Source: three-view drawing plus pictorial views. Frame: mm from the lowest corner of the part. A direction names the side the tool comes from. Give positions to 0.01 mm unless a question says otherwise; leave off trailing zeros. Loops run counter-clockwise (first coordinate to the right, second up) from the corner with the lowest first, then second, coordinate; pieces in that order, holes last. Notation, with made-up numbers: (43.25, -30) -> (68.25, -30) arc R19 cw to (68.25, 4) -> close; hole circle Ø7 at (14.5, 10). An arc over 180 degrees is marked (long way). Answer in a Markdown table with one row per item. Add a question column.
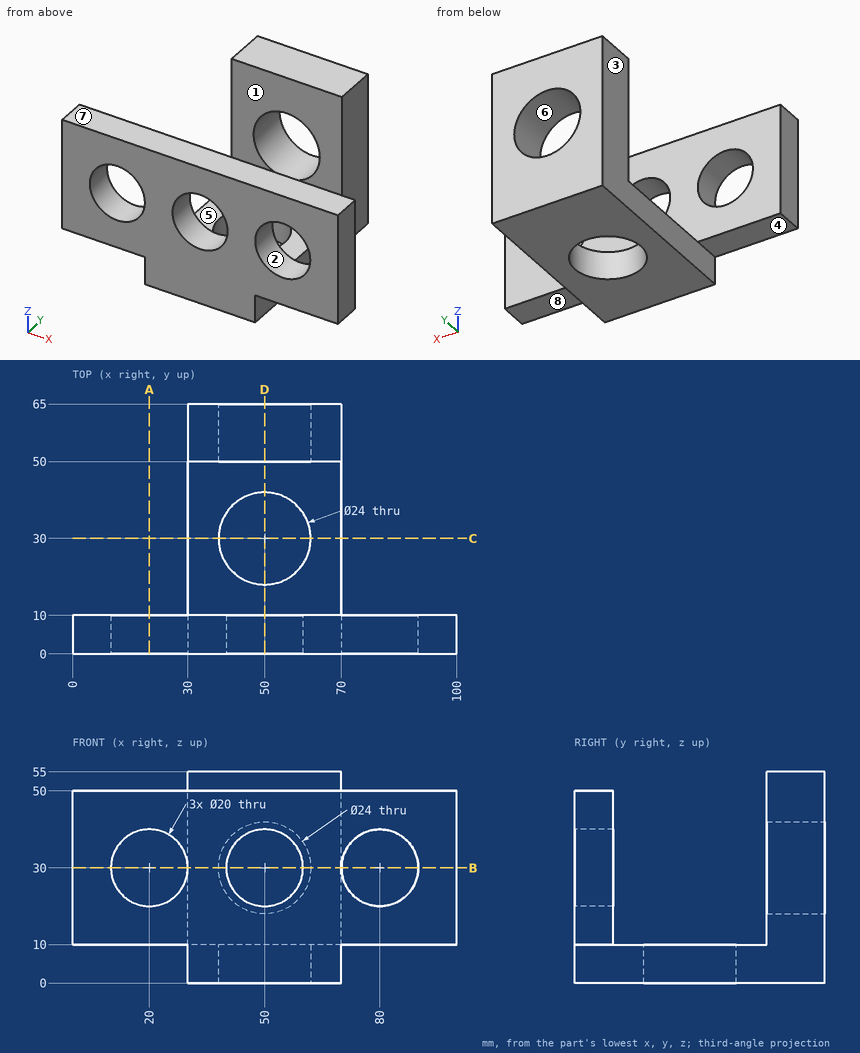
(1) Cut plane C-C on y = 30. Return the cut outline in (x, z).
(2) Reachability of the marked faces 4, 5, 6, 7 and 8 from +Z, -Z, +X, -X, +Y, -Y: full face, straight path, thin tool, end or side. Return the list, or none.
(3) Cut plane B-B on z = 30. Return the cut outline in (x, y), then the cut area to 3 significant figures.
(4) Draft query along X for the marked faces 1, 2 and 3. Return one class per face: +X half, -X half, draft (parallel to the pull), parting line (faces both ways), or undercut.
(5) Pin query (flat end, axial travel): pin 1 Ø11 at (x, y) = (15, 3.5) entering from -Z; pin 2 Ø1.5 at (y, z) = (24.5, 10) entering from -X; pin 3 Ø2 at (x, z) = (71.5, 9.5) entering from +Y. Return the tip coordinate at first contact, or that it passes through.
(6) Cut plane A-A on x = 20. Return the cut outline in (y, z).
(7) Material intervals for line 1 along X through (y, z) = (61.5, 29.5); line 2 along Y through (x, z) = (56, 40.5); line 3 along Y through (x, z) = (50, 5.25), sorted ascending. Write a range as from..to.
(8) Cut plane D-D on x = 50. Return the cut outline in (y, z), then the cut area to 3 significant figures.
Answer list:
| question | item | result |
|---|---|---|
| 1 | outline | (30, 0) -> (38, 0) -> (38, 10) -> (30, 10) -> close; (62, 0) -> (70, 0) -> (70, 10) -> (62, 10) -> close |
| 2 | face 4 | -Z, -X, +Y, -Y |
| 2 | face 5 | +Z, +X, -X |
| 2 | face 6 | +Y |
| 2 | face 7 | +Z, +X, -X, -Y |
| 2 | face 8 | -Z, +X, +Y, -Y |
| 3 | outline | (0, 0) -> (10, 0) -> (10, 10) -> (0, 10) -> close; (30, 0) -> (40, 0) -> (40, 10) -> (30, 10) -> close; (30, 50) -> (38, 50) -> (38, 65) -> (30, 65) -> close; (60, 0) -> (70, 0) -> (70, 10) -> (60, 10) -> close; (62, 50) -> (70, 50) -> (70, 65) -> (62, 65) -> close; (90, 0) -> (100, 0) -> (100, 10) -> (90, 10) -> close |
| 3 | area | 640 mm² |
| 4 | face 1 | draft |
| 4 | face 2 | undercut |
| 4 | face 3 | -X half |
| 5 | pin 1 | stops at z = 10 |
| 5 | pin 2 | stops at x = 30 |
| 5 | pin 3 | stops at y = 10 |
| 6 | outline | (0, 10) -> (10, 10) -> (10, 20) -> (0, 20) -> close; (0, 40) -> (10, 40) -> (10, 50) -> (0, 50) -> close |
| 7 | line 1 | x = 30..38.01, 61.99..70 |
| 7 | line 2 | y = 0..10, 50..65 |
| 7 | line 3 | y = 0..18, 42..65 |
| 8 | outline | (0, 0) -> (18, 0) -> (18, 10) -> (10, 10) -> (10, 20) -> (0, 20) -> close; (0, 40) -> (10, 40) -> (10, 50) -> (0, 50) -> close; (42, 0) -> (65, 0) -> (65, 18) -> (50, 18) -> (50, 10) -> (42, 10) -> close; (50, 42) -> (65, 42) -> (65, 55) -> (50, 55) -> close |
| 8 | area | 925 mm² |
